Autodesk Fusion 360 part; units mm, degrees
sketch "Sketch1" plane through (0, 0, 0) normal (0, 1, 0) x (1, 0, 0)
  circle A0 centre (0, 0) radius 40
  circle A1 centre (0, 0) radius 37
  dimension "d1" = 80
  dimension "d7" = 3
extrude "Extrude1" add sketch "Sketch1" along normal blind 100 makes body 1
extrude "Extrude2" add sketch "Sketch1" along normal blind 4 contours A1 bodies 1
copy_body "Body->Comp1" bodies 1 removing the originals makes body 2 in component "tubeToolHolder05"
component "tubeToolHolder05" placed x (1, 0, 0) y (0, 1, 0) z (0, 0, 1) at (0, 0, 0)
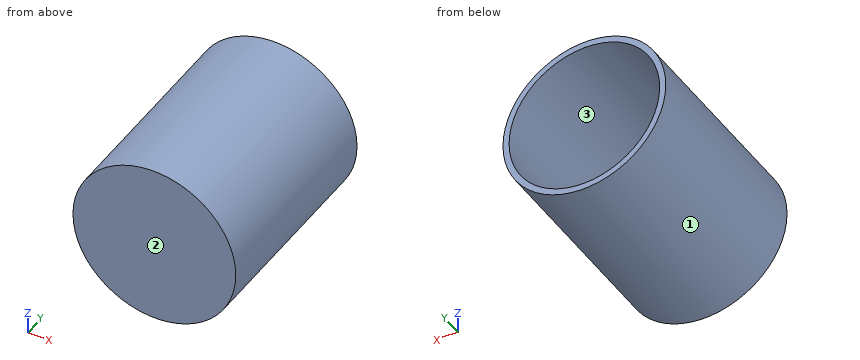
Source: CAD feature listing. Evaluate the final solid. Frame: model axes, mm. Face numbers are marked on the shaded views. Give positions to 0.01 mm unless a question says otherwise; leave off trailing zeros. Write each loop counter-clockwise with the first axis right and the second up, starting at its lowest first coordinate (ties: lowest second). Pieces come first, ordered by that corner, then holes. Notation, with made-up numbers: (75, 85.5) -> (113, 85.5) arc R20 ccw to (113, 116.5) -> close; hole circle Ø3 at (28, 70). An arc over 180 degrees is marked (long way). Return JSON: item names as keys, results as strings. Group by question number.
1. Mould query, pull axis Z, two halves, no side actions, for the marked faces 1, 2 and 3. Classes: +Z half, -Z half, draft (parallel to the pull), parting line (faces both ways), or undercut.
2. Section C-C, the plane y = 87.5. Output: boundary loops of the cut face in (x, z).
3. Section A-A, the plane x = 0. Output: boundary loops of the cut face in (y, z).
4. Material intervals for line 1 (Z direction, x = 0, y = 74); line 2 (Y direction, x = -25.5, z = -18.5), sorted ascending. Write a range as from..to.
5. Section B-B, the plane z = 0. Output: boundary loops of the cut face in (x, y), then the cut area to 3 significant figures.
6. Pin query (flat end, axial travel): pin 1 Ø5 at (x, y) = (27, 19) entering from -Z; pin 2 Ø2 at (x, y) = (8, 72) entering from -Z; pin 3 Ø3 at (y, z) = (52, -29) entering from -X. Return the tip coordinate at first contact, or that it passes through.
Determined:
{
 "1": {"face 1": "parting line", "face 2": "draft", "face 3": "undercut"},
 "2": {"outline": "circle Ø80 at (0, 0); hole circle Ø74 at (0, 0)"},
 "3": {"outline": "(0, -40) -> (100, -40) -> (100, -37) -> (4, -37) -> (4, 37) -> (100, 37) -> (100, 40) -> (0, 40) -> close"},
 "4": {"line 1": "z = -40..-37, 37..40", "line 2": "y = 0..4"},
 "5": {"outline": "(-40, 0) -> (40, 0) -> (40, 100) -> (37, 100) -> (37, 4) -> (-37, 4) -> (-37, 100) -> (-40, 100) -> close", "area": "896 mm2"},
 "6": {"pin 1": "stops at z = -31.62", "pin 2": "stops at z = -39.38", "pin 3": "stops at x = -29.05"}
}
